CAD build for the part. Positions are in the model's coordinates, mm. A direction names the side the tool comes from. Coordinates: 2 decimals unless noted, no trailing zeros. Order: outer loops, then holes, each group sorted by start corner. A loop starts at its lowest first (then second) coordinate and runs counter-clockwise, first axis right, second up. Notation, with made-up numbers: M 75.5,8 L 97.5,8 A31 ccw 97.5,44 Z; hole C -37,52.5 d8. An arc over 180 degrees is marked long. Write item = value, one per line. Start each with the question number.
```python
from build123d import *

# Parameters (mm, degrees)
F1_DEPTH = 10
F2_W     = 10
F2_H     = 10
F3_DEPTH = 10


with BuildPart() as f1:
    # F0 (on Top) → F1 (new body)
    with BuildSketch(Plane.XY):
        Polygon((-16.419269, 6.361689), (-16.419269, 6.013863), (-16.419269, -13.638311), (13.580731, -13.638311), (13.580731, 6.361689), (3.580731, 6.361689), (3.580731, -3.638311), (-6.419269, -3.638311), (-6.419269, 6.361689), align=None)
    extrude(amount=F1_DEPTH)

    # F2 (on face) → F3 (join)
    with BuildSketch(Plane.XY.offset(10)):
        with Locations((-11.419269, 1.361689)):
            Rectangle(F2_W, F2_H)
    extrude(amount=F3_DEPTH)


solid = f1.part
```
1. Slice it at C-C (x = -12.5). Write the cut outline in (y, z).
2. Slice it at B-B (z = 8.75). Write the cut outline in (x, y).
3. Flat gauge pins, fed straight in: pin 1 (5 mm diameter, centred on x = 0.5, z = 7.5, fed in from +Y); pin 2 (2 mm diameter, centred on x = -5.5, y = -8.5, fed in from +Z); pin 3 (11 mm diameter, centred on x = -12, z = 16.5, fed in from -Y). Where does each tip first touch, or does it go through?
4. Mould opens along X. For faces 4 (the flat face through (3.581, 1, 5)), 5 (the flat face through (-1, -3.638, 5)), 6 (the flat face through (-11, -3.638, 15)), 7 (the flat face through (13.581, -4, 5)) say: released by +X, released by -X, zero draft, split by the parting line, or undercut.
5. Slice it at D-D (y = -4.5). Write the cut outline in (x, z), plus the area to 3 significant figures.
6. Slice it at A-A (y = 0.5). Write the cut outline in (x, z).
7. 3-axis set-ups, long thin cutter, end or side, ignore diameter. For faces 1 (the flat face through (-6.419, 1, 10)), 2 (the flat face through (2, -6, 10)), 3 (the flat face through (-11, 6.362, 10)): which of +Z, -Z, +X, -X, +Y, -Y reach the whole face in a straight line?
8. Probe L1, parallel to X at y = -2, z = 5.5; L2, parallel to Z at x = -2, y = -6; L3, parallel to Y at x = -9, z = 10.75. List the from-to ranges inside material, lowest first.
Calculated:
q1.outline = M -13.64,0 L 6.36,0 L 6.36,20 L -3.64,20 L -3.64,10 L -13.64,10 Z
q2.outline = M -16.42,-13.64 L 13.58,-13.64 L 13.58,6.36 L 3.58,6.36 L 3.58,-3.64 L -6.42,-3.64 L -6.42,6.36 L -16.42,6.36 Z
q3.pin_1 = -3.64
q3.pin_2 = 10
q3.pin_3 = -3.64
q4.face_4 = undercut
q4.face_5 = undercut
q4.face_6 = zero draft
q4.face_7 = released by +X
q5.outline = M -16.42,0 L 13.58,0 L 13.58,10 L -16.42,10 Z
q5.area = 300 mm²
q6.outline = M -16.42,0 L -6.42,0 L -6.42,20 L -16.42,20 Z; M 3.58,0 L 13.58,0 L 13.58,10 L 3.58,10 Z
q7.face_1 = +Z, -Z, +Y
q7.face_2 = +Z, +X, -Y
q7.face_3 = +Z, -Z, +X, -X, +Y
q8.L1 = -16.42 to -6.42, 3.58 to 13.58
q8.L2 = 0 to 10
q8.L3 = -3.64 to 6.36
